Verification items for this drawing (mm, ordinates from the low corner). A direction names the side the tool comes from. Give positions to 0.01 mm unless a question says otherwise; leave off trailing zeros. Order: outer loops, then holes, each group sorted by start corner. A loop starts at its lowest first (then second) coordinate and runs counter-clockwise, first axis right, second up. Notation, with made-up numbers: M -15.5,-25.5 L 10.5,-25.5 A34 cw 10.5,13.5 Z; hole C -9,-36 d1. An arc over 180 degrees is marked long. One line per question, with ' | ' between items. Start each with the question number.
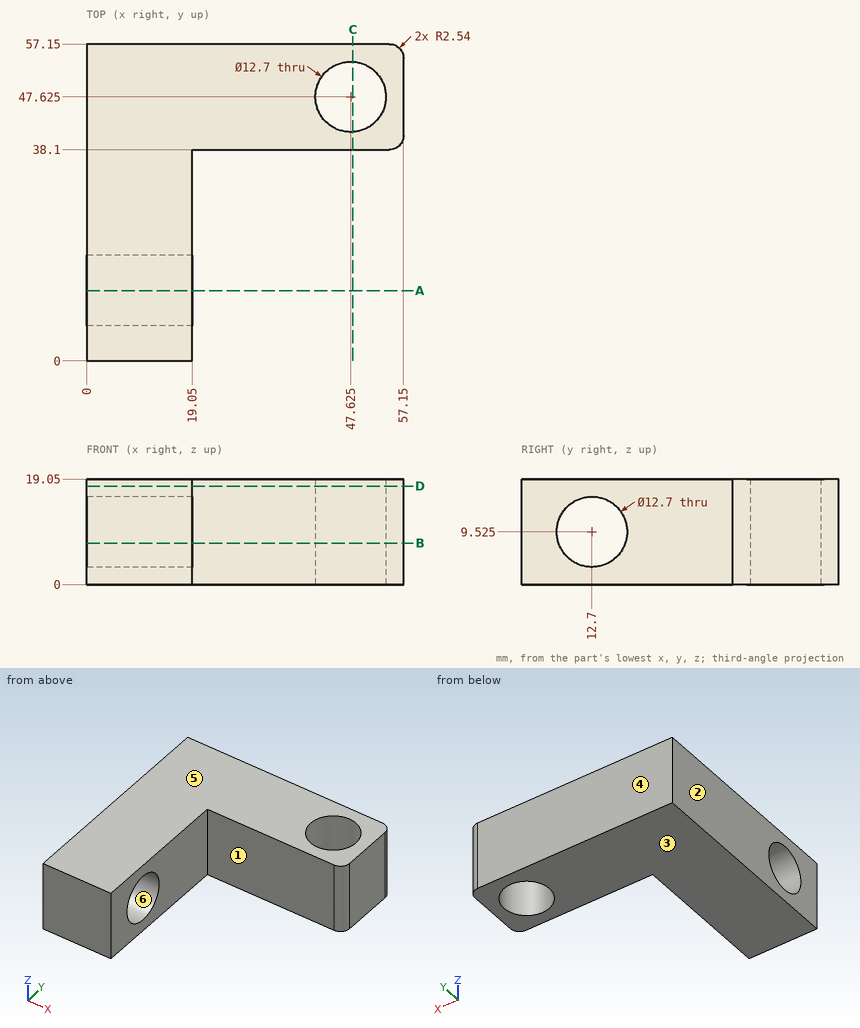
Item 1: Cross-section at B-B, the plane z = 7.5. Record the cut outline in (x, y) (3 decimals).
Item 2: Depth check by flat-ended pin: pin 1 (2 mm diameter, centred on x = 25.5, z = 13.5, fed in from -Y); pin 2 (9.5 mm diameter, centred on y = 18, z = 7, fed in from +X); pin 3 (14.5 mm diameter, centred on x = 47.625, y = 47.625, fed in from -Z). Enter the tip coordinate at first touch or a pass-through.
Item 3: Cross-section at C-C, the plane x = 48. Record the cut outline in (y, z), plus the area to 3 significant figures.
Item 4: Cross-section at A-A, the plane y = 12.7. Record the cut outline in (x, z) (3 decimals).
Item 5: Cross-section at D-D, the plane z = 17.75. Record the cut outline in (x, y) (3 decimals), plus the area to 3 significant figures.
Item 6: Set-up check for the marked faces 1 and 2: record each of +Z, -Z, +X, -X, +Y, -Y from which the full face is reachable in a straight line by a thin tool's end or side.
Item 7: Mould release check, pull along Z, two halves, no side actions. Record for the marked faces 3, 4, 5 and 6: released by +Z, released by -Z, zero draft, split by the parting line, or undercut.
Item 8: Material ranges on line 1 along Z through (x, y) = (14.5, 12.7) (3 decimals); line 2 along X through (y, z) = (34, 7.75), recorded low to high.
Outcome:
1) outline: M 0,0 L 19.05,0 L 19.05,6.682 L 0,6.682 Z; M 0,18.718 L 19.05,18.718 L 19.05,38.1 L 54.61,38.1 A2.54 ccw 57.15,40.64 L 57.15,54.61 A2.54 ccw 54.61,57.15 L 0,57.15 Z; hole C 47.625,47.625 d12.7
2) pin 1: stops at y = 38.1 | pin 2: stops at x = 19.05 | pin 3: stops at z = 0
3) outline: M 38.1,0 L 41.29,0 L 41.29,19.05 L 38.1,19.05 Z; M 53.96,0 L 57.15,0 L 57.15,19.05 L 53.96,19.05 Z | area: 121 mm²
4) outline: M 0,0 L 19.05,0 L 19.05,3.175 L 0,3.175 Z; M 0,15.875 L 19.05,15.875 L 19.05,19.05 L 0,19.05 Z
5) outline: M 0,0 L 19.05,0 L 19.05,38.1 L 54.61,38.1 A2.54 ccw 57.15,40.64 L 57.15,54.61 A2.54 ccw 54.61,57.15 L 0,57.15 Z; hole C 47.625,47.625 d12.7 | area: 1,690 mm²
6) face 1: +Z, -Z, +X, -Y | face 2: +Z, -Z, -X, +Y, -Y
7) face 3: released by -Z | face 4: zero draft | face 5: released by +Z | face 6: undercut
8) line 1: z = 0 to 3.175, 15.875 to 19.05 | line 2: x = 0 to 19.05
